Can you work these out from the model? Positions are in its coordinate system, mm. Give positions to 0.01 mm unless a question says otherwise; leave off trailing zeros. Write each loop counter-clockwise with the first axis right and the second up, starting at its lowest first coordinate (ties: lowest second). Pieces come first, ordered by that corner, then holes.
from build123d import *

# Parameters (mm, degrees)
SKETCH1_R           = 3.175
BOSS_EXTRUDE1_DEPTH = 2.54
SKETCH2_R           = 2.38125
CUT_EXTRUDE1_DEPTH  = 3.54
SKETCH5_R           = 2.5527
CUT_EXTRUDE2_DEPTH  = 3.54
SKETCH6_R           = 2.38125
SKETCH6_R_2         = 14.1605
CUT_EXTRUDE3_DEPTH  = 3.54
SKETCH7_R           = 14.1605
SKETCH7_R_2         = 2.38125
BOSS_EXTRUDE2_DEPTH = 2.54
SKETCH8_R           = 14.2875
CUT_EXTRUDE4_DEPTH  = 3.54


with BuildPart() as part:
    # Sketch1 → Boss-Extrude1 (new body)
    with BuildSketch(Plane(origin=(2097.33945945, 0, 0), x_dir=(0, 0, -1), z_dir=(1, 0, 0))):
        with BuildLine():
            Line((470.462593133, 294.283973481), (380.69060226, -25.250155611))
            ThreePointArc((380.69060226, -25.250155611), (396.988966218, -67.7453513), (442.372216694, -64.304580962))
            Line((442.372216694, -64.304580962), (633.066836095, -65.629031002))
            ThreePointArc((633.066836095, -65.629031002), (637.543938621, -67.520043059), (639.372580729, -72.022980064))
            Line((639.372580729, -72.022980064), (638.556689771, -189.495146754))
            ThreePointArc((638.556689771, -189.495146754), (640.385331878, -193.998083759), (644.862434405, -195.889095816))
            Line((644.862434405, -195.889095816), (816.308299304, -197.079855594))
            Line((816.308299304, -197.079855594), (819.660067566, 285.508504864))
            ThreePointArc((819.660067566, 285.508504864), (817.831425459, 290.01144187), (813.354322932, 291.902453927))
            Line((813.354322932, 291.902453927), (470.462593133, 294.283973481))
        make_face()
        with Locations((553.895503221, -55.553924847)):
            Circle(SKETCH1_R, mode=Mode.SUBTRACT)
        with Locations((738.492000758, 61.775645376)):
            Circle(SKETCH1_R, mode=Mode.SUBTRACT)
        with Locations((779.099930223, -68.570323835)):
            Circle(SKETCH1_R, mode=Mode.SUBTRACT)
        with Locations((654.585392145, -186.431395895)):
            Circle(SKETCH1_R, mode=Mode.SUBTRACT)
        with Locations((417.370503221, -35.55524491)):
            Circle(SKETCH1_R, mode=Mode.SUBTRACT)
        with Locations((629.958065992, -56.082209622)):
            Circle(SKETCH1_R, mode=Mode.SUBTRACT)
    extrude(amount=BOSS_EXTRUDE1_DEPTH)

    # Sketch2 → Cut-Extrude1 (cut, through all)
    with BuildSketch(Plane(origin=(2099.87945945, 0, 0), x_dir=(0, 0, -1), z_dir=(1, 0, 0))):
        with Locations((759.618090186, -100.982485439)):
            Circle(SKETCH2_R)
        with Locations((541.187693092, 46.53204311)):
            Circle(SKETCH2_R)
        with Locations((478.851639869, 34.42970992)):
            Circle(SKETCH2_R)
        with Locations((416.515586647, 22.327376731)):
            Circle(SKETCH2_R)
        with Locations((525.320503221, -14.245042905)):
            Circle(SKETCH2_R)
        with Locations((798.886947172, 37.479390763)):
            Circle(SKETCH2_R)
        with Locations((665.859799537, 70.736709489)):
            Circle(SKETCH2_R)
        with Locations((603.523746314, 58.634376299)):
            Circle(SKETCH2_R)
        with Locations((703.559149884, -143.519538535)):
            Circle(SKETCH2_R)
        with Locations((726.384244699, -115.392244277)):
            Circle(SKETCH2_R)
        with Locations((804.898658391, -11.249556635)):
            Circle(SKETCH2_R)
        with Locations((474.520503221, -14.245042905)):
            Circle(SKETCH2_R)
        with Locations((651.589984927, -141.551336746)):
            Circle(SKETCH2_R)
        with Locations((651.589984927, -90.751336746)):
            Circle(SKETCH2_R)
        with Locations((593.128456503, -52.651336746)):
            Circle(SKETCH2_R)
    extrude(amount=-CUT_EXTRUDE1_DEPTH, mode=Mode.SUBTRACT)

    # Sketch5 → Cut-Extrude2 (cut, through all)
    with BuildSketch(Plane(origin=(2099.87945945, 0, 0), x_dir=(0, 0, -1), z_dir=(1, 0, 0))):
        with Locations((395.373457964, -48.255244909)):
            Circle(SKETCH5_R)
        with Locations((405.46425322, -56.177474835)):
            Circle(SKETCH5_R)
        with Locations((395.373457964, -22.855244907)):
            Circle(SKETCH5_R)
        with Locations((393.55800322, -35.555244908)):
            Circle(SKETCH5_R)
        with Locations((417.370503221, -10.155244906)):
            Circle(SKETCH5_R)
        with Locations((405.46425322, -14.93301498)):
            Circle(SKETCH5_R)
        with Locations((439.367548478, -22.855244907)):
            Circle(SKETCH5_R)
        with Locations((429.276753221, -14.93301498)):
            Circle(SKETCH5_R)
        with Locations((439.367548478, -48.255244909)):
            Circle(SKETCH5_R)
        with Locations((441.183003221, -35.555244908)):
            Circle(SKETCH5_R)
        with Locations((417.370503221, -60.955244909)):
            Circle(SKETCH5_R)
        with Locations((429.276753221, -56.177474835)):
            Circle(SKETCH5_R)
    extrude(amount=-CUT_EXTRUDE2_DEPTH, mode=Mode.SUBTRACT)

    # Sketch6 → Cut-Extrude3 (cut, through all)
    with BuildSketch(Plane.ZY.offset(-2099.87945945)):
        with Locations((-714.213403899, 41.676013157)):
            Circle(SKETCH6_R)
        with Locations((-714.213403899, 77.597201157)):
            Circle(SKETCH6_R)
        with Locations((-732.173834383, 85.036607157)):
            Circle(SKETCH6_R)
        with Locations((-750.134264867, 77.597201157)):
            Circle(SKETCH6_R)
        with Locations((-750.134264867, 41.676013157)):
            Circle(SKETCH6_R)
        with Locations((-732.173834383, 34.236607157)):
            Circle(SKETCH6_R)
        with Locations((-732.173834383, 59.636607157)):
            Circle(SKETCH6_R_2)
    extrude(amount=CUT_EXTRUDE3_DEPTH, mode=Mode.SUBTRACT)

    # Sketch7 → Boss-Extrude2 (add)
    with BuildSketch(Plane(origin=(2099.87945945, 0, 0), x_dir=(0, 0, -1), z_dir=(1, 0, 0))):
        with Locations((732.173834383, 59.636607157)):
            Circle(SKETCH7_R)
        with Locations((732.173834383, 59.636607157)):
            Circle(SKETCH7_R_2, mode=Mode.SUBTRACT)
    extrude(amount=-BOSS_EXTRUDE2_DEPTH)

    # Sketch8 → Cut-Extrude4 (cut, through all)
    with BuildSketch(Plane.ZY.offset(-2097.33945945)):
        with Locations((-732.173834383, 59.636607157)):
            Circle(SKETCH8_R)
        with Locations((-779.099930223, -68.570323835)):
            Circle(SKETCH8_R)
    extrude(amount=-CUT_EXTRUDE4_DEPTH, mode=Mode.SUBTRACT)


solid = part.part
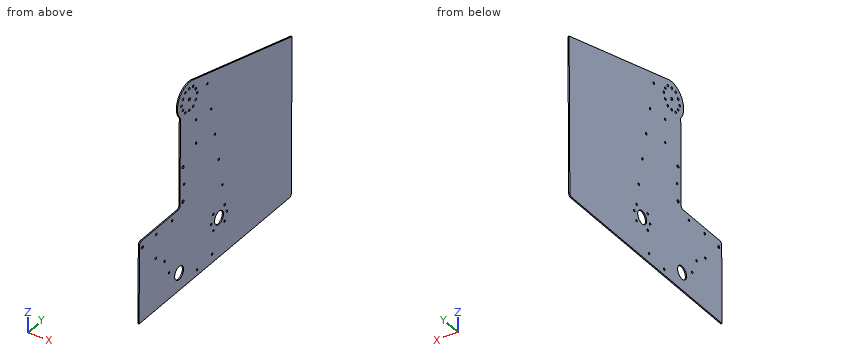
(1) Imagine slicing it at C-C, the plane z = -618. Write out the boundary of the cut face in (x, y), plus the area to 3 significant figures.
Returned:
outline: (2097.34, -65.52) - (2099.88, -65.52) - (2099.88, 293.26) - (2097.34, 293.26) - close
area: 911 mm2
(2) Imagine slicing it at B-B, the plane x = 2098.55. Give the number of separate pieces and of enclosed holes in the cut face, plus the area to 3 significant figures.
Returned:
separate pieces: 1
enclosed holes: 39
area: 164,000 mm2
(3) If I drill on L1, parallel to Z at x = 2098.8, y = 77; L2, parallel to Z at x = 2099.75, y = -59; L3, parallel to Z at x = 2097.5, y = 60, over which ranges is the centre line in solid material (lowest first)?
Returned:
L1: z = -818.21 to -752.44, -747.83 to -716.52, -711.91 to -409.42
L2: z = -817.27 to -789.71, -768.49 to -631.21, -628.71 to -419.01, -415.73 to -387.34
L3: z = -818.09 to -746.46, -717.89 to -605.47, -601.57 to -404.64
(4) Imagine slicing it at A-A, the plane y = 239.5. Write out the boundary of the cut face in (x, z).
Returned:
outline: (2097.34, -819.34) - (2099.88, -819.34) - (2099.88, -455.07) - (2097.34, -455.07) - close
(5) Will these pins go through, and if not, where does the flat tip stop? P1, Ø4.5, axis at y = 70.74, z = -665.86, coming from the -X side; P2, Ø1.5, axis at x = 2099, z = -608.5, coming from the -Y side.
Returned:
P1: passes through
P2: stops at y = -65.46
